For this review, take the finished solid that the model builds, in its own axes (mm). A direction names the side the tool comes from. Round coordinates to 2 decimals unless told otherwise and drop trailing zeros. Write each loop counter-clockwise with the first axis right and the second up, starting at its lowest first coordinate (ties: lowest second). Pieces come first, ordered by that corner, then holes. Notation, with made-up numbers: M -5.75,86 L 18.25,86 A27 ccw 18.25,114 Z; hole C 17,47 d8. An arc over 180 degrees is marked long. Use one line per item in the form item = value. Start each with the question number.
Item 1: Add section A-A (z = 2.8). State the section outline as (x, y) points, and give its area (3 significant figures).
Item 2: Draft analysis for pull direction Y (two halves, no side actions). For faces 1 (the flat face through (-34, 12, -1)), 2 (the cylindrical face through (33.6, 5.8, 5.1)), 3 (the flat face through (-34, 0, -1)), state which applies: released by +Y, released by -Y, zero draft, split by the parting line, or undercut.
Item 3: For faces 4 (the flat face through (0, 9, 32)), 5 (the cylindrical face through (-16.603, 6.09, -36.549)), 6 (the flat face through (-1, 6, -40)), 7 (the cylindrical face through (-0.499, 3.505, 36.056)), list the 3-axis set-ups (+Z, -Z, +X, -X, +Y, -Y) from which the entire face can be reached by the end or side of a thin tool; tool diameter is ignored.
Item 4: Add section D-D (y = 10). State the section outline as (x, z) points.
Item 5: Add section C-C (z = -13). State the section outline as (x, y) points, and give its area (3 significant figures).
Item 6: Add section B-B (x = -19.5). State the section outline as (y, z) points, and give its area (3 significant figures).
Item 7: For P1, Ø3.5, axis at x = 0, y = 5.75, coming from the +Z side, flat-tipped, find the tip position at first contact; note if it passes through.
Item 8: For line 1 (X direction, y = 10.5, z = 7.5); line 2 (Z direction, x = -1.5, y = 9.75); line 3 (Y direction, x = 33.5, z = 2.8), list the stretches that pass through material, from the lowest coordinate up. Write a range as [from, to].
from build123d import *

# Parameters (mm, degrees)
SKETCH1_W           = 75
SKETCH1_H           = 80
BOSS_EXTRUDE1_DEPTH = 12
SKETCH2_W           = 59
SKETCH2_H           = 65
CUT_EXTRUDE1_DEPTH  = 11
SKETCH3_W           = 55
SKETCH3_H           = 63
CUT_EXTRUDE2_DEPTH  = 56.921820428
SKETCH5_R           = 2.9
CUT_EXTRUDE4_DEPTH  = 7
SKETCH7_W           = 57
SKETCH7_H           = 64
CUT_EXTRUDE5_DEPTH  = 56.921820428
SKETCH9_R           = 2.3
CUT_EXTRUDE6_DEPTH  = 8
SKETCH10_R          = 2.3
CUT_EXTRUDE7_DEPTH  = 86.842879728


with BuildPart() as part:
    # Sketch1 → Boss-Extrude1 (new body)
    with BuildSketch(Plane(origin=(0, 0, 0), x_dir=(1, 0, 0), z_dir=(0, 1, 0))):
        Rectangle(SKETCH1_W, SKETCH1_H)
    extrude(amount=BOSS_EXTRUDE1_DEPTH)

    # Sketch2 → Cut-Extrude1 (cut)
    with BuildSketch(Plane(origin=(0, 12, 0), x_dir=(1, 0, 0), z_dir=(0, 1, 0))):
        with Locations((0, 0.5)):
            Rectangle(SKETCH2_W, SKETCH2_H)
    extrude(amount=-CUT_EXTRUDE1_DEPTH, mode=Mode.SUBTRACT)

    # Sketch3 → Cut-Extrude2 (cut, through all)
    with BuildSketch(Plane(origin=(0, 1, 0), x_dir=(1, 0, 0), z_dir=(0, 1, 0))):
        with Locations((0, 1.5)):
            Rectangle(SKETCH3_W, SKETCH3_H)
    extrude(amount=-CUT_EXTRUDE2_DEPTH, mode=Mode.SUBTRACT)

    # Sketch5 → Cut-Extrude4 (cut)
    with BuildSketch(Plane(origin=(0, 0, -40), x_dir=(-1, 0, 0), z_dir=(0, 0, -1))):
        with Locations((-19.5, 5.962429795)):
            Circle(SKETCH5_R)
        with Locations((19.5, 5.962429795)):
            Circle(SKETCH5_R)
    extrude(amount=-CUT_EXTRUDE4_DEPTH, mode=Mode.SUBTRACT)

    # Sketch7 → Cut-Extrude5 (cut, through all)
    with BuildSketch(Plane(origin=(0, 1, 0), x_dir=(1, 0, 0), z_dir=(0, 1, 0))):
        with Locations((0, 1)):
            Rectangle(SKETCH7_W, SKETCH7_H)
    extrude(amount=-CUT_EXTRUDE5_DEPTH, mode=Mode.SUBTRACT)

    # Sketch9 → Cut-Extrude6 (cut)
    with BuildSketch(Plane.XY.offset(40)):
        with Locations((0, 5.75)):
            Circle(SKETCH9_R)
    extrude(amount=-CUT_EXTRUDE6_DEPTH, mode=Mode.SUBTRACT)

    # Sketch10 → Cut-Extrude7 (cut, through all)
    with BuildSketch(Plane(origin=(37.5, 0, 0), x_dir=(0, 0, -1), z_dir=(1, 0, 0))):
        with Locations((-2.8, 5.719569138)):
            Circle(SKETCH10_R)
    extrude(amount=-CUT_EXTRUDE7_DEPTH, mode=Mode.SUBTRACT)


solid = part.part
Calculated:
q1.outline = M -37.5,0 L -28.5,0 L -28.5,1 L -29.5,1 L -29.5,3.42 L -37.5,3.42 Z; M -37.5,8.02 L -29.5,8.02 L -29.5,12 L -37.5,12 Z; M 28.5,0 L 37.5,0 L 37.5,3.42 L 29.5,3.42 L 29.5,1 L 28.5,1 Z; M 29.5,8.02 L 37.5,8.02 L 37.5,12 L 29.5,12 Z
q1.area = 120 mm^2
q2.face_1 = released by +Y
q2.face_2 = undercut
q2.face_3 = released by -Y
q3.face_4 = +Y
q3.face_5 = -Z
q3.face_6 = -Z, +X, -X, +Y, -Y
q3.face_7 = +Z
q4.outline = M -37.5,-40 L 37.5,-40 L 37.5,40 L -37.5,40 Z; hole M -29.5,-33 L 29.5,-33 L 29.5,32 L -29.5,32 Z
q5.outline = M -37.5,0 L -28.5,0 L -28.5,1 L -29.5,1 L -29.5,12 L -37.5,12 Z; M 28.5,0 L 37.5,0 L 37.5,12 L 29.5,12 L 29.5,1 L 28.5,1 Z
q5.area = 194 mm^2
q6.outline = M 0,-40 L 3.06,-40 L 3.06,-33 L 0,-33 Z; M 0,31 L 1,31 L 1,32 L 12,32 L 12,40 L 0,40 Z; M 8.86,-40 L 12,-40 L 12,-33 L 8.86,-33 Z
q6.area = 140 mm^2
q7.P1 = -33
q8.line_1 = [-37.5, -29.5], [29.5, 37.5]
q8.line_2 = [-40, -33], [32, 40]
q8.line_3 = [0, 3.42], [8.02, 12]
